from build123d import *

# Parameters (mm, degrees)
SKETCH2_R          = 4
CUT_EXTRUDE1_DEPTH = 27.697325265
SKETCH3_R          = 1.5
CUT_EXTRUDE2_DEPTH = 27.697325265
SKETCH4_R          = 1.5
CUT_EXTRUDE3_DEPTH = 27.697325352


with BuildPart() as part:
    # Sketch1 → Revolve1 (revolve)
    with BuildSketch(Plane(origin=(0, 0, 0), x_dir=(1, 0, 0), z_dir=(0, 1, 0)), mode=Mode.PRIVATE) as revolve1_sk:
        Polygon((0, 23), (-5.9, 23), (-5.9, 13), (-9.585071109, 13), (-9.585071109, 12), (-8.085071109, 12), (-8.085071109, 1), (-9.585071109, 1), (-9.585071109, 0), (0, 0), align=None)
    revolve(revolve1_sk.sketch.rotate(Axis((0, 0, 0), (0, 0, -1)), 180), axis=Axis((0, 0, 0), (0, 0, -1)))

    # Sketch2 → Cut-Extrude1 (cut, through all)
    with BuildSketch(Plane.XY):
        Circle(SKETCH2_R)
    extrude(amount=-CUT_EXTRUDE1_DEPTH, mode=Mode.SUBTRACT)

    # Sketch3 → Cut-Extrude2 (cut, through all)
    with BuildSketch(Plane(origin=(0, 0, 0), x_dir=(1, 0, 0), z_dir=(0, 1, 0))):
        with Locations(Location((0, 18, 0), (0, 0, 270))):
            Circle(SKETCH3_R)
    extrude(amount=-CUT_EXTRUDE2_DEPTH, mode=Mode.SUBTRACT)

    # Sketch4 → Cut-Extrude3 (cut, through all)
    with BuildSketch(Plane(origin=(0, 0, 0), x_dir=(0, 0, -1), z_dir=(1, 0, 0))):
        with Locations((18, 0)):
            Circle(SKETCH4_R)
    extrude(amount=-CUT_EXTRUDE3_DEPTH, mode=Mode.SUBTRACT)


solid = part.part
Read the model definition and answer for the solid it produces. Units are mm, in the model's axes. A direction names the side the tool comes from. Round coordinates to 2 decimals unless told otherwise and drop trailing zeros. Loops run counter-clockwise (first coordinate to the right, second up) from the corner with the lowest first, then second, coordinate; pieces in that order, holes last.
Q1. Section C-C on x = 3 is taken. Write down the section's boundary in (y, z).
Q2. Each of these flat-tipped pins is pushed along its axis until it touches: pin 1 (10 mm diameter, centred on x = 1, y = -1.5, fed in from +Z); pin 2 (4 mm diameter, centred on x = 1, z = -4.5, fed in from -Y); pin 3 (3 mm diameter, centred on y = -5, z = -8, fed in from -X); pin 4 (1 mm diameter, centred on y = 5, z = -2.5, fed in from +X). Where does it stop, or does it pass through?
Q3. Section D-D on z = -10 is taken. Write down the section's boundary in (x, y).
Q4. Which of the six approach directions +Z, -Z, +X, -X, +Y, -Y give full straight-line access (tool end or side, diameter ignored) to faces 5 (the face through (-4.79, 0.07, -16.5)), 6 (the face through (-2.078, 9.357, -0.493)), 7 (the face through (-4.3, 7.1, -12)), 8 (the face through (2.722, 5.234, -17.93)), 9 (the face through (0.07, -4.79, -19.5))?
Q5. Determine the mould class of faces 1 (the face through (2, 4, 0)), 2 (the face through (0.1, 6.3, -13)), 3 (the face through (7.71, -2.43, -6.42)), 4 (the face through (4.3, 7.1, -1)) for opening direction Z: released by +Z, released by -Z, zero draft, split by the parting line, or undercut.
Q6. Section A-A on y = 0 is taken. Write down the section's boundary in (x, z), and give its area (3 significant figures).
Q7. Consider probe 1 along Z at (x, y) = (0.25, -8.5); probe 2 along Y at (x, z) = (0, -13.25); probe 3 along Z at (x, y) = (0, -5). Determine where each line is inside the solid, lowest interval first.
Output:
1. outline: (-9.1, -13) - (-5.08, -13) - (-5.08, -23) - (-2.65, -23) - (-2.65, 0) - (-9.1, 0) - (-9.1, -1) - (-7.51, -1) - (-7.51, -12) - (-9.1, -12) - close; (2.65, -23) - (5.08, -23) - (5.08, -13) - (9.1, -13) - (9.1, -12) - (7.51, -12) - (7.51, -1) - (9.1, -1) - (9.1, 0) - (2.65, 0) - close
2. pin 1: stops at z = 0
2. pin 2: stops at y = -8.09
2. pin 3: stops at x = -7.29
2. pin 4: stops at x = 6.72
3. outline: circle Ø16.17 at (0, 0); hole circle Ø8 at (0, 0)
4. face 5: -X
4. face 6: +Z, -Z
4. face 7: none
4. face 8: -Z
4. face 9: -Y
5. face 1: released by +Z
5. face 2: released by -Z
5. face 3: undercut
5. face 4: undercut
6. outline: (-9.59, -13) - (-5.9, -13) - (-5.9, -16.5) - (-4, -16.5) - (-4, 0) - (-9.59, 0) - (-9.59, -1) - (-8.09, -1) - (-8.09, -12) - (-9.59, -12) - close; (-5.9, -23) - (-4, -23) - (-4, -19.5) - (-5.9, -19.5) - close; (4, -23) - (5.9, -23) - (5.9, -13) - (9.59, -13) - (9.59, -12) - (8.09, -12) - (8.09, -1) - (9.59, -1) - (9.59, 0) - (4, 0) - close
6. area: 145 mm2
7. probe 1: z = -13 to -12, -1 to 0
7. probe 2: y = -5.9 to -4, 4 to 5.9
7. probe 3: z = -23 to -19.5, -16.5 to 0
